from build123d import *

# Parameters (mm, degrees)
BOSS_EXTRUDE1_DEPTH = 7
CHAMFER1_SIZE       = 1.5


with BuildPart() as part:
    # Sketch1 → Boss-Extrude1 (new body)
    with BuildSketch(Plane(origin=(0, 0, 0), x_dir=(1, 0, 0), z_dir=(0, 1, 0))):
        with BuildLine():
            Line((-29.2, 3.8), (-28.878460969, 5))
            Line((-28.878460969, 5), (0, 5))
            ThreePointArc((0, 5), (5, 0), (0, -5))
            Line((0, -5), (-28.878460969, -5))
            Line((-28.878460969, -5), (-29.2, -3.8))
            Line((-29.2, -3.8), (-30, -3.8))
            Line((-30, -3.8), (-30, -7.2))
            Line((-30, -7.2), (0, -7.2))
            ThreePointArc((0, -7.2), (7.2, 0), (0, 7.2))
            Line((0, 7.2), (-30, 7.2))
            Line((-30, 7.2), (-30, 3.8))
            Line((-30, 3.8), (-29.2, 3.8))
        make_face()
    extrude(amount=BOSS_EXTRUDE1_DEPTH)

    # Chamfer1
    chamfer1_edges = [part.edges().sort_by_distance(p)[0] for p in [
        (-30, 3.5, -7.2),
        (-30, 3.5, 7.2),
    ]]
    chamfer(chamfer1_edges, length=CHAMFER1_SIZE)


solid = part.part
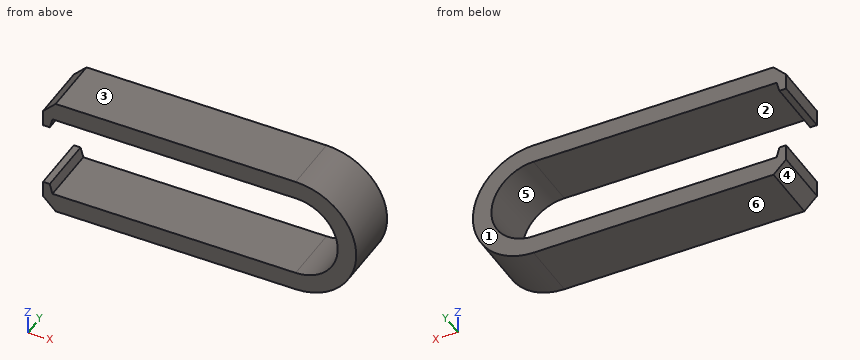
Geometry check sheet. Reference: the model listing, model coordinates, mm. Face numbers are marked on the shaded views. A direction names the side the tool comes from. Round coordinates to 2 decimals unless told otherwise and drop trailing zeros. Order: outer loops, then holes, each group sorted by start corner. A loop starts at its lowest first (then second) coordinate and runs counter-clockwise, first axis right, second up. Notation, with made-up numbers: (-18.75, 65) - (38.25, 65) arc R11 cw to (38.25, 83) - close; hole circle Ø3 at (-5, 69.5). An arc over 180 degrees is marked (long way). One line per question, with ' | ' between items. Start each with the question number.
(1) Sectioned sample at B-B on y = 0.5. Record the cut outline in (x, z), and give its area (3 significant figures).
(2) Thickness scan on L1, parallel to Z at x = -3.5, y = 5.5; L2, parallel to X at y = 5.5, z = -4.5; L3, parallel to Z at x = 1.5, y = 3.5. Record the ranges inside material, lowest first. Write a range as [from, to].
(3) Sectioned sample at A-A on x = -14. Record the cut outline in (y, z).
(4) Release check for a two-part mould opening along Z. For the marked faces 1, 2, 3 and 4 record: released by +Z, released by -Z, zero draft, split by the parting line, or undercut.
(5) Depth check by flat-ended pin: pin 1 Ø1 at (y, z) = (1, -3.5) entering from +X; pin 2 Ø0.9 at (x, y) = (-29.5, 2) entering from +Z. Enter the tip coordinate at first touch or a pass-through.
(6) Sectioned sample at D-D on z = 3. Record the cut outline in (x, y), and give its area (3 significant figures).
(7) Sectioned sample at C-C on z = 0. Record the cut outline in (x, y).
(8) Access from +Z, -Z, +X, -X, +Y, -Y to the whole of each face (thin tool, end or side, straight path). Record for the marked faces 5 and 6.
Conclusion:
1) outline: (-30, -5.7) - (-28.5, -7.2) - (0, -7.2) arc R7.2 ccw to (0, 7.2) - (-28.5, 7.2) - (-30, 5.7) - (-30, 3.8) - (-29.2, 3.8) - (-28.88, 5) - (0, 5) arc R5 cw to (0, -5) - (-28.88, -5) - (-29.2, -3.8) - (-30, -3.8) - close | area: 174 mm2
2) L1: z = [-7.2, -5], [5, 7.2] | L2: x = [-30, -29.01], [2.18, 5.62] | L3: z = [-7.04, -4.77], [4.77, 7.04]
3) outline: (0, -7.2) - (7, -7.2) - (7, -5) - (0, -5) - close; (0, 5) - (7, 5) - (7, 7.2) - (0, 7.2) - close
4) face 1: zero draft | face 2: undercut | face 3: released by +Z | face 4: released by -Z
5) pin 1: stops at x = 6.55 | pin 2: stops at z = 6.65
6) outline: (4, 0) - (6.55, 0) - (6.55, 7) - (4, 7) - close | area: 17.8 mm2
7) outline: (5, 0) - (7.2, 0) - (7.2, 7) - (5, 7) - close
8) face 5: +Y, -Y | face 6: -Z, +X, -X, +Y, -Y
